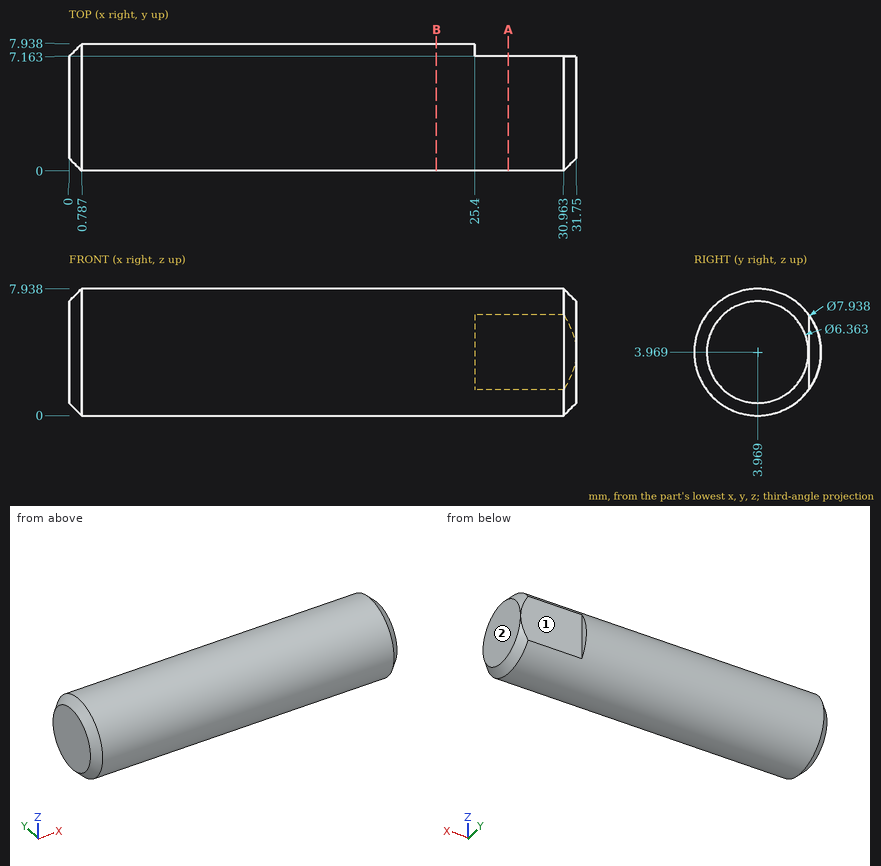
Print and shaded views of the part. All mm, measured from the part's lowest x, y and z. A direction names the side the tool comes from. Give positions to 0.01 mm unless a question says otherwise; leave off trailing zeros. Write each loop counter-clockwise with the first axis right and the second up, starting at its lowest first coordinate (ties: lowest second). Pieces come first, ordered by that corner, then holes. Notation, with made-up numbers: (56.25, 16) -> (114.25, 16) arc R19 cw to (114.25, 50) -> close; hole circle Ø10 at (4, 81). An arc over 180 degrees is marked (long way). Write item = value, one per line.
(1) Flat gauge pins, fed straight in: P1, Ø2, axis at x = 19, y = 6, coming from the +Z side; P2, Ø2, axis at x = 9.5, z = 2.5, coming from the +Y side; P3, Ø0.6, axis at y = 7.5, z = 3.5, coming from the +X side. Where does each tip first touch, or does it go through?
Determined:
P1 = 7.8
P2 = 7.91
P3 = 25.4
(2) Tool access for the marked faces 1 and 2: list every direction of +Z, -Z, +X, -X, +Y, -Y with a clear straight run to the whole face (end or side of a thin tool).
Determined:
face_1 = +Z, -Z, +X, +Y
face_2 = +Z, -Z, +X, +Y, -Y
(3) Slice it at A-A, the plane x = 27.5. Give the cut face in (y, z) (1 decimal), then the cut area to 3 significant figures.
Determined:
outline = (7.2, 1.6) -> (7.2, 6.3) arc R4 ccw (long way) to start
area = 47.0 mm2
(4) Slice it at B-B, the plane x = 23. Give the cut face in (y, z).
Determined:
outline = circle Ø7.94 at (3.97, 3.97)
(5) Probe line 1 along X through (y, z) = (3, 7); line 2 along Y through (x, z) = (12, 4.75); line 3 along Z through (x, y) = (7, 3.25) (1 decimal). List the from-to ranges inside material, lowest first.
Determined:
line_1 = 0 to 31.75
line_2 = 0.08 to 7.86
line_3 = 0.1 to 7.9
